Check sheet for the modelled part. Datum: model origin and axes. Units: mm. Face numbers are marked on the shaded views. A direction names the side the tool comes from. Coordinates: 2 decimals unless noted, no trailing zeros. Order: outer loops, then holes, each group sorted by start corner. A loop starts at its lowest first (then second) coordinate and runs counter-clockwise, first axis right, second up. Notation, with made-up numbers: (19.25, 36.25) -> (57.25, 36.25) arc R21 ccw to (57.25, 47.25) -> close; hole circle Ø10 at (82.25, -37.75). An arc over 180 degrees is marked (long way). Put each result on its own line as item: value. Start each with the question number.
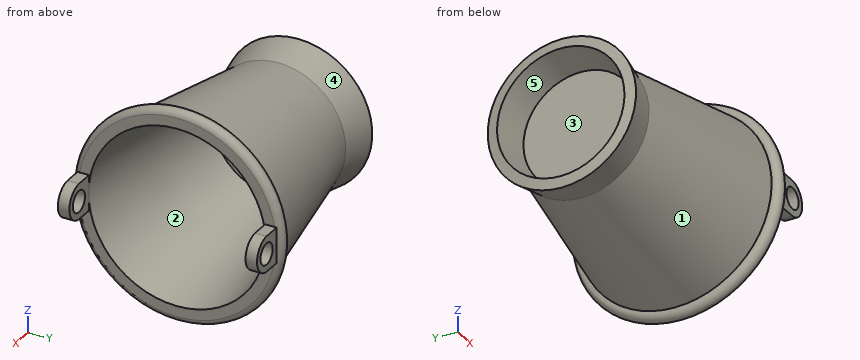
```python
from build123d import *

# Parameters (mm, degrees)
SKETCH2_W           = 5
SKETCH2_H           = 1.623250271
BOSS_EXTRUDE1_DEPTH = 5
CUT_EXTRUDE1_DEPTH  = 26.500274
SKETCH4_R           = 1.5
CUT_EXTRUDE2_DEPTH  = 26.500274


with BuildPart() as part:
    # Sketch1 → Revolve1 (revolve)
    with BuildSketch(Plane(origin=(0, 0, 0), x_dir=(1, 0, 0), z_dir=(0, 1, 0))):
        with BuildLine():
            Line((1.257722515, 9.518975428), (24.380809012, 13.648394277))
            ThreePointArc((24.380809012, 13.648394277), (25.189431543, 14.808622531), (26.349659797, 14))
            Line((26.349659797, 14), (26.349659797, 12.5))
            Line((26.349659797, 12.5), (2.479732811, 8.649095646))
            Line((2.479732811, 8.649095646), (2.479732811, 0))
            Line((2.479732811, 0), (0.979732811, 0))
            Line((0.979732811, 0), (0.979732811, 8.0625))
            Line((0.979732811, 8.0625), (-3.931590203, 9))
            Line((-3.931590203, 9), (-3.650340203, 10.473396904))
            Line((-3.650340203, 10.473396904), (1.257722515, 9.518975428))
        make_face()
    revolve(axis=Axis((-20.81402906, 0, 0), (1, 0, 0)))

    # Sketch2 → Boss-Extrude1 (add)
    with BuildSketch(Plane(origin=(26.349659797, 0, 0), x_dir=(0, 0, -1), z_dir=(1, 0, 0))):
        with Locations((0, 13.250136984)):
            Rectangle(SKETCH2_W, SKETCH2_H)
        with Locations((0, -13.250136984)):
            Rectangle(SKETCH2_W, SKETCH2_H)
    extrude(amount=BOSS_EXTRUDE1_DEPTH)

    # Sketch3 → Cut-Extrude1 (cut)
    with BuildSketch(Plane(origin=(0, 14.061762119, 0), x_dir=(1, 0, 0), z_dir=(0, 1, 0))):
        with BuildLine():
            Line((28.849659797, 2.5), (31.349659797, 2.5))
            Line((31.349659797, 2.5), (31.349659797, -2.5))
            Line((31.349659797, -2.5), (28.849659797, -2.5))
            ThreePointArc((28.849659797, -2.5), (31.217194374, 0), (28.849659797, 2.5))
        make_face()
    cut_extrude1 = extrude(amount=-CUT_EXTRUDE1_DEPTH, mode=Mode.SUBTRACT)

    # Mirror1: Cut-Extrude1 across plane
    add(cut_extrude1.mirror(Plane.ZX), mode=Mode.SUBTRACT)

    # Sketch4 → Cut-Extrude2 (cut)
    with BuildSketch(Plane(origin=(0, 14.061762119, 0), x_dir=(1, 0, 0), z_dir=(0, 1, 0))):
        with Locations((28.849659797, 0)):
            Circle(SKETCH4_R)
    cut_extrude2 = extrude(amount=-CUT_EXTRUDE2_DEPTH, mode=Mode.SUBTRACT)

    # Mirror2: Cut-Extrude2 across plane
    add(cut_extrude2.mirror(Plane.ZX), mode=Mode.SUBTRACT)


solid = part.part
```
1) Sectioned sample at A-A (z = 0). State how many separate pieces and enclosed holes the cut face has, plus the area to 3 significant figures.
2) Access from +Z, -Z, +X, -X, +Y, -Y to the whole of each face (thin tool, end or side, straight path). Record for the marked faces 4 and 5.
3) Gauge pin test, flat ends, axial feed: pin 1 (2 mm diameter, centred on x = 13, y = 0.5, fed in from +Z); pin 2 (14 mm diameter, centred on y = -1.5, z = 10, fed in from +X); pin 3 (0.5 mm diameter, centred on x = 27, y = -13.5, fed in from -Z); pin 4 (12 mm diameter, centred on y = 3, z = -7.5, fed in from -X). Record the tip position at first contact, or that the pin passes through.
4) Mould release check, pull along Z, two halves, no side actions. Record for the marked faces 1, 2 and 3: +Z half, -Z half, draft (parallel to the pull), parting line (faces both ways), or undercut.
5) Scan lines: line 1 along Y through (x, z) = (27, -1.5); line 2 along Y through (x, z) = (19.5, 2.5); line 3 along Z through (x, y) = (5, 0). Record each from-to range of solid material in increasing order. Write a range as [from, to].
6) Sectioned sample at C-C (x = 0.5). Record the boundary of the cut face in (y, z).
7) Sectioned sample at D-D (x = 12). Record the boundary of the cut face in (y, z), plus the area to 3 significant figures.
8) Sectioned sample at B-B (y = 0). Record the boundary of the cut face in (x, z), plus the area to 3 significant figures.
Entries:
1. separate pieces: 3
1. enclosed holes: 0
1. area: 114 mm2
2. face 4: none
2. face 5: -X
3. pin 1: stops at z = 11.79
3. pin 2: stops at x = 26.35
3. pin 3: stops at z = -2.5
3. pin 4: stops at x = -3.93
4. face 1: parting line
4. face 2: undercut
4. face 3: undercut
5. line 1: y = [-14.06, -12.44], [12.44, 14.06]
5. line 2: y = [-12.53, -11.12], [11.12, 12.53]
5. line 3: z = [-10.19, -9.06], [9.06, 10.19]
6. outline: circle Ø19.33 at (0, 0); hole circle Ø16.31 at (0, 0)
7. outline: circle Ø22.87 at (0, 0); hole circle Ø20.37 at (0, 0)
7. area: 85.1 mm2
8. outline: (-3.93, -9) -> (-3.65, -10.47) -> (1.26, -9.52) -> (24.38, -13.65) arc R1 ccw to (26.35, -14) -> (26.35, -12.5) -> (2.48, -8.65) -> (2.48, 8.65) -> (26.35, 12.5) -> (26.35, 14) arc R1 ccw to (24.38, 13.65) -> (1.26, 9.52) -> (-3.65, 10.47) -> (-3.93, 9) -> (0.98, 8.06) -> (0.98, -8.06) -> close
8. area: 108 mm2
